Build history of the part. All positions in model axes, mm. A direction names the side the tool comes from. Give positions to 0.01 mm unless a question says otherwise; leave off trailing zeros. Order: outer loops, then holes, each group sorted by start corner. A loop starts at its lowest first (then second) coordinate and runs counter-clockwise, first axis right, second up. Notation, with made-up numbers: M 14.25,47.5 L 26.25,47.5 A9 cw 26.25,59.5 Z; hole C -30.5,57 d8. An arc over 180 degrees is marked long. One line per item, written item: value.
from build123d import *

# Parameters (mm, degrees)
SKETCH1_W           = 53.34
SKETCH1_H           = 158.75
SKETCH1_R           = 1
BOSS_EXTRUDE1_DEPTH = 6.35
SKETCH2_W           = 31.75
SKETCH2_H           = 6.35
BOSS_EXTRUDE2_DEPTH = 31.75
SKETCH3_W           = 31.75
SKETCH3_H           = 6.35
BOSS_EXTRUDE3_DEPTH = 12.7
CUT_EXTRUDE1_REACH  = 143.732
SKETCH4_R           = 12.573
SKETCH5_W           = 31.75
SKETCH5_H           = 2.671239047
SKETCH5_H_2         = 2.428760953
BOSS_EXTRUDE4_DEPTH = 6.35
FILLET1_R           = 5.08


with BuildPart() as part:
    # Sketch1 → Boss-Extrude1 (new body)
    with BuildSketch(Plane.XY):
        with Locations((-17.091445783, 49.935481928)):
            Rectangle(SKETCH1_W, SKETCH1_H)
        with Locations((-36.141445783, 69.620481928)):
            Circle(SKETCH1_R, mode=Mode.SUBTRACT)
        with Locations((-8.201445783, 69.620481928)):
            Circle(SKETCH1_R, mode=Mode.SUBTRACT)
        with Locations((-41.221445783, 121.690481928)):
            Circle(SKETCH1_R, mode=Mode.SUBTRACT)
        with Locations((7.038554217, 120.420481928)):
            Circle(SKETCH1_R, mode=Mode.SUBTRACT)
    extrude(amount=BOSS_EXTRUDE1_DEPTH)

    # Sketch2 → Boss-Extrude2 (add)
    with BuildSketch(Plane.XY.offset(6.35)):
        with Locations((-17.091445783, 60.014063864)):
            Rectangle(SKETCH2_W, SKETCH2_H)
    extrude(amount=BOSS_EXTRUDE2_DEPTH)

    # Sketch3 → Boss-Extrude3 (add)
    with BuildSketch(Plane(origin=(0, 63.189063864, 0), x_dir=(1, 0, 0), z_dir=(0, 1, 0))):
        with Locations((-17.091445783, -34.925)):
            Rectangle(SKETCH3_W, SKETCH3_H)
    extrude(amount=BOSS_EXTRUDE3_DEPTH)

    # Sketch4 → Cut-Extrude1 (cut, up to next)
    with BuildSketch(Plane.XY.offset(38.1), mode=Mode.PRIVATE) as cut_extrude1_sk1:
        with Locations((-17.091445783, 78.510481928)):
            Circle(SKETCH4_R)
    cut_extrude1_tool1 = extrude(cut_extrude1_sk1.sketch, amount=-CUT_EXTRUDE1_REACH, mode=Mode.PRIVATE) & part.part
    add(cut_extrude1_tool1.solids().sort_by_distance((-17.091446, 78.510482, 38.1))[0], mode=Mode.SUBTRACT)

    # Sketch5 → Boss-Extrude4 (add)
    with BuildSketch(Plane(origin=(0, 63.189063864, 0), x_dir=(1, 0, 0), z_dir=(0, 1, 0))):
        with Locations((-17.091445783, -33.085619524)):
            Rectangle(SKETCH5_W, SKETCH5_H)
        with Locations((-17.091445783, -36.885619523)):
            Rectangle(SKETCH5_W, SKETCH5_H_2)
    extrude(amount=BOSS_EXTRUDE4_DEPTH)

    # Fillet1
    fillet1_edges = [part.edges().sort_by_distance(p)[0] for p in [
        (-17.091445783, 63.189063864, 31.75),
    ]]
    fillet(fillet1_edges, radius=FILLET1_R)


solid = part.part
1) Saw through at D-D, the plane y = 96. Write the cut outline in (x, z).
Check values:
outline: M -43.76,0 L 9.58,0 L 9.58,6.35 L -43.76,6.35 Z
2) Saw through at A-A, the plane y = 61. Write the cut outline in (x, z).
Check values:
outline: M -43.76,0 L 9.58,0 L 9.58,6.35 L -1.22,6.35 L -1.22,38.1 L -32.97,38.1 L -32.97,6.35 L -43.76,6.35 Z
3) Saw through at C-C, the plane z = 20.5. Write the cut outline in (x, y), then the cut area to 3 significant figures.
Check values:
outline: M -32.97,56.84 L -1.22,56.84 L -1.22,63.19 L -32.97,63.19 Z
area: 202 mm^2
4) Drill centre lines: probe 1 along Z at (x, y) = (-19, 68.5); probe 2 along Z at (x, y) = (-15, 87); probe 3 along Y at (x, z) = (-5, 8). Where is each one in solid material? Low to high. Write a range as from..to.
Check values:
probe 1: 0..6.35, 31.75..34.42, 35.67..38.1
probe 2: 0..6.35
probe 3: 56.84..63.19
5) Mould opens along X. For faces 4 (the face through (-31, 75.889, 35)), 5 (the face through (-17, 69.539, 33)), 6 (the face through (-43.761, 49, 3)) say: released by +X, released by -X, zero draft, split by the parting line, or undercut.
Check values:
face 4: zero draft
face 5: undercut
face 6: released by -X
6) Tool access for faces 1 (the face through (-17, 68, 34.421)), 2 (the face through (-17, 63.189, 16)), 3 (the face through (-1.216, 62, 26)): list every direction of +Z, -Z, +X, -X, +Y, -Y with a clear straight run to the whole face (end or side of a thin tool).
Check values:
face 1: +Y
face 2: +X, -X, +Y
face 3: +Z, +X, +Y, -Y
7) Saw through at B-B, the plane x = -19. Write the cut outline in (y, z), then the cut area to 3 significant figures.
Check values:
outline: M -29.44,0 L 129.31,0 L 129.31,6.35 L 63.19,6.35 L 63.19,26.67 A5.08 cw 68.27,31.75 L 69.54,31.75 L 69.54,34.42 L 66.08,34.42 L 66.08,35.67 L 69.54,35.67 L 69.54,38.1 L 56.84,38.1 L 56.84,6.35 L -29.44,6.35 Z
area: 1,250 mm^2
8) Pin check, flat tips, straight feed: pin 1 (1.8 mm diameter, centred on x = -41.22, y = 121.69, fed in from -Z); pin 2 (1 mm diameter, centred on x = -3, z = 17.5, fed in from -Y); pin 3 (2 mm diameter, centred on x = -16.5, z = 32.5, fed in from +Y); pin 4 (6 mm diameter, centred on x = -10, z = 20.5, fed in from +Y). Stop position of each tip, or through.
Check values:
pin 1: through
pin 2: y = 56.84
pin 3: y = 69.54
pin 4: y = 63.19
